```python
from build123d import *

# Parameters (mm, degrees)
SKETCH1_W           = 23
SKETCH1_H           = 104.5
SKETCH1_R           = 2
SKETCH1_R_2         = 5.2
BOSS_EXTRUDE1_DEPTH = 5
SKETCH2_W           = 23
SKETCH2_H           = 20
BOSS_EXTRUDE2_DEPTH = 20
SKETCH3_W           = 23
SKETCH3_H           = 20
BOSS_EXTRUDE3_DEPTH = 5
SKETCH3_3_W         = 100
SKETCH3_3_H         = 20
BOSS_EXTRUDE4_DEPTH = 10
BOSS_EXTRUDE5_DEPTH = 30
BOSS_EXTRUDE6_DEPTH = 30
FILLET1_R           = 10
CUT_EXTRUDE1_DEPTH  = 300
SKETCH6_R           = 13.5
CUT_EXTRUDE2_DEPTH  = 162.5
FILLET5_R           = 3


with BuildPart() as part:
    # Sketch1 → Boss-Extrude1 (new body)
    with BuildSketch(Plane.XY):
        with Locations((0, 30.75)):
            Rectangle(SKETCH1_W, SKETCH1_H)
        with Locations((6.5, 16.5)):
            Circle(SKETCH1_R, mode=Mode.SUBTRACT)
        with Locations((6.5, -16.5)):
            Circle(SKETCH1_R, mode=Mode.SUBTRACT)
        with Locations((0, -12)):
            Circle(SKETCH1_R_2, mode=Mode.SUBTRACT)
        with Locations((-6.5, -16.5)):
            Circle(SKETCH1_R, mode=Mode.SUBTRACT)
        with Locations((-6.5, 16.5)):
            Circle(SKETCH1_R, mode=Mode.SUBTRACT)
    extrude(amount=BOSS_EXTRUDE1_DEPTH)

    # Sketch2 → Boss-Extrude2 (add)
    with BuildSketch(Plane(origin=(0, 0, 0), x_dir=(-1, 0, 0), z_dir=(0, 0, -1))):
        with Locations((0, 73)):
            Rectangle(SKETCH2_W, SKETCH2_H)
    extrude(amount=BOSS_EXTRUDE2_DEPTH)

    # Sketch3 → Boss-Extrude3 (add)
    with BuildSketch(Plane(origin=(0, 0, -20), x_dir=(-1, 0, 0), z_dir=(0, 0, -1))):
        with Locations((0, 73)):
            Rectangle(SKETCH3_W, SKETCH3_H)
    extrude(amount=BOSS_EXTRUDE3_DEPTH)

    # Sketch3<3> → Boss-Extrude4 (add)
    with BuildSketch(Plane(origin=(0, 0, -20), x_dir=(-1, 0, 0), z_dir=(0, 0, -1))):
        with Locations((-61.5, 73)):
            Rectangle(SKETCH3_3_W, SKETCH3_3_H)
        with Locations((61.5, 73)):
            Rectangle(SKETCH3_3_W, SKETCH3_3_H)
    extrude(amount=BOSS_EXTRUDE4_DEPTH)

    # Sketch4 → Boss-Extrude5 (add)
    with BuildSketch(Plane(origin=(111.5, 0, 0), x_dir=(0, 0, -1), z_dir=(1, 0, 0))):
        with BuildLine():
            Line((30, 83), (30, 79.422616289))
            ThreePointArc((30, 79.422616289), (37.803170415, 82.465987391), (44.982034231, 78.151420148))
            Line((44.982034231, 78.151420148), (47.256120501, 79.619062793))
            ThreePointArc((47.256120501, 79.619062793), (39.346969169, 84.978803601), (30, 83))
        make_face()
        with BuildLine():
            ThreePointArc((44.982034231, 67.848579852), (37.803170415, 63.534012609), (30, 66.577383711))
            Line((30, 66.577383711), (30, 63))
            ThreePointArc((30, 63), (39.346969169, 61.021196399), (47.256120501, 66.380937207))
            Line((47.256120501, 66.380937207), (44.982034231, 67.848579852))
        make_face()
    extrude(amount=-BOSS_EXTRUDE5_DEPTH)

    # Sketch5 → Boss-Extrude6 (add)
    with BuildSketch(Plane.ZY.offset(111.5)):
        with BuildLine():
            ThreePointArc((-44.99074033, 78.15631214), (-37.806835348, 82.471571982), (-30, 79.42472441))
            Line((-30, 79.42472441), (-30, 82.742901835))
            ThreePointArc((-30, 82.742901835), (-39.236660525, 84.790740062), (-47.086393259, 79.50952476))
            Line((-47.086393259, 79.50952476), (-44.99074033, 78.15631214))
        make_face()
        with BuildLine():
            Line((-30, 63.257098165), (-30, 66.57527559))
            ThreePointArc((-30, 66.57527559), (-37.806835348, 63.528428018), (-44.99074033, 67.84368786))
            Line((-44.99074033, 67.84368786), (-47.086393259, 66.49047524))
            ThreePointArc((-47.086393259, 66.49047524), (-39.236660525, 61.209259938), (-30, 63.257098165))
        make_face()
    extrude(amount=-BOSS_EXTRUDE6_DEPTH)

    # Fillet1
    fillet1_edges = [part.edges().sort_by_distance(p)[0] for p in [
        (11.5, 73, -20),
        (-11.5, 73, -20),
    ]]
    fillet(fillet1_edges, radius=FILLET1_R)

    # Sketch4<3> → Cut-Extrude1 (cut)
    with BuildSketch(Plane(origin=(111.5, 0, 0), x_dir=(0, 0, -1), z_dir=(1, 0, 0))):
        with BuildLine():
            Line((30, 66.577383711), (30, 73))
            Line((30, 73), (27.5, 73))
            ThreePointArc((27.5, 73), (28.147034395, 69.553987812), (30, 66.577383711))
        make_face()
        with BuildLine():
            Line((27.5, 73), (30, 73))
            Line((30, 73), (30, 79.422616289))
            ThreePointArc((30, 79.422616289), (28.147034395, 76.446012188), (27.5, 73))
        make_face()
    extrude(amount=-CUT_EXTRUDE1_DEPTH, mode=Mode.SUBTRACT)

    # Sketch6 → Cut-Extrude2 (cut)
    with BuildSketch(Plane(origin=(-81.5, 0, 0), x_dir=(0, 0, -1), z_dir=(1, 0, 0))):
        with Locations((37.005416749, 73)):
            Circle(SKETCH6_R)
    extrude(amount=CUT_EXTRUDE2_DEPTH, mode=Mode.SUBTRACT)

    # Fillet5
    # the kernel refuses this fillet: 3 mm, written as the material it takes off along each edge
    with BuildSketch(Plane(origin=(118.086652749, 67.848579852, -44.982034231), x_dir=(0, -0.768500975054365, 0.6398486159557513), z_dir=(-1, 0, 0))) as fillet5_piece_1:
        with BuildLine():
            CenterArc((2.659503922, -2.977998992), FILLET5_R, 96.943270181, 76.113459637)
            Line((-0.318495069, -2.615339366), (-0.378055049, -2.608086174))
            Line((-0.378055049, -2.608086174), (-0.05955998, 0.007253193))
            Line((-0.05955998, 0.007253193), (0.007253193, 0.05955998))
            ThreePointArc((0.007253193, 0.05955998), (1.148422148, -0.009669859), (2.289591104, 0.05955998))
            Line((2.289591104, 0.05955998), (2.296844297, 0))
        make_face()
    extrude(amount=43.173305498, mode=Mode.SUBTRACT)
    with BuildSketch(Plane(origin=(-117.736458127, 67.84368786, -44.99074033), x_dir=(0, -0.5424603966463132, -0.8400813758620795), z_dir=(1, 0, 0))) as fillet5_piece_2:
        with BuildLine():
            CenterArc((2.635643587, -2.996681829), FILLET5_R, 92.695047673, 73.440207037)
            Line((-0.276948751, -2.277789714), (-0.335200598, -2.263411872))
            ThreePointArc((-0.335200598, -2.263411872), (-0.129052561, -1.140040424), (-0.06, 0))
            Line((-0.06, 0), (0, 0.06))
            ThreePointArc((0, 0.06), (1.247291625, 0.06), (2.491762044, 0.059933637))
            Line((2.491762044, 0.059933637), (2.494583251, 0))
        make_face()
    extrude(amount=42.472916254, mode=Mode.SUBTRACT)
    with BuildSketch(Plane(origin=(-117.736458127, 78.15631214, -44.99074033), x_dir=(0, 0.7684660550632233, 0.6398905548729151), z_dir=(1, 0, 0))) as fillet5_piece_3:
        with BuildLine():
            CenterArc((2.656657786, -2.978067915), FILLET5_R, 96.932372645, 73.440207037)
            Line((-0.301090552, -2.476346114), (-0.360245519, -2.466311678))
            ThreePointArc((-0.360245519, -2.466311678), (-0.210106634, -1.230931193), (-0.059561358, 0.007241864))
            Line((-0.059561358, 0.007241864), (0.007241864, 0.059561358))
            ThreePointArc((0.007241864, 0.059561358), (1.147282288, -0.009491202), (2.287322712, 0.059561358))
            Line((2.287322712, 0.059561358), (2.294564576, 0))
        make_face()
    extrude(amount=42.472916254, mode=Mode.SUBTRACT)
    with BuildSketch(Plane(origin=(118.086652749, 78.151420148, -44.982034231), x_dir=(0, 0.5422547524206679, -0.8402141295391314), z_dir=(-1, 0, 0))) as fillet5_piece_4:
        with BuildLine():
            CenterArc((2.6346611, -3), FILLET5_R, 90, 76.113459637)
            Line((-0.277657564, -2.28), (-0.335903938, -2.2656))
            ThreePointArc((-0.335903938, -2.2656), (-0.129229839, -1.141168956), (-0.06, 0))
            Line((-0.06, 0), (0, 0.06))
            Line((0, 0.06), (2.6346611, 0.06))
            Line((2.6346611, 0.06), (2.6346611, 0))
        make_face()
    extrude(amount=43.173305498, mode=Mode.SUBTRACT)


solid = part.part
```
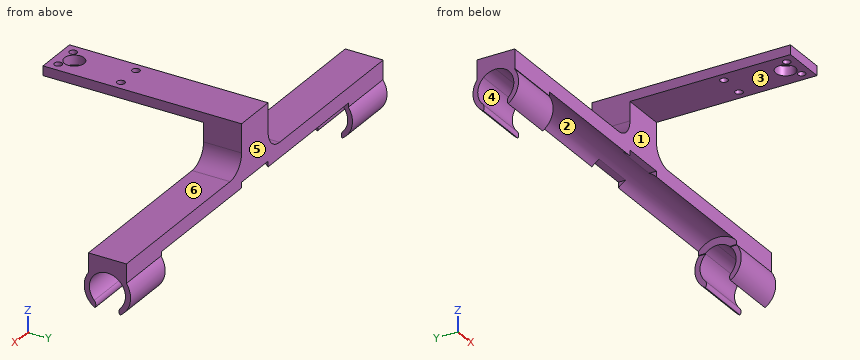
Here's how the part is built. I have some questions about the finished solid (model axes, mm). Face numbers are marked on the shaded views. A direction names the side the tool comes from. Round coordinates to 2 decimals unless told otherwise and drop trailing zeros. Write each loop counter-clockwise with the first axis right and the second up, starting at its lowest first coordinate (ties: lowest second). Pieces come first, ordered by that corner, then holes. Notation, with made-up numbers: M 26.5,81 L 76.5,81 A30 ccw 76.5,112 Z; hole C -20,21.5 d8. An arc over 180 degrees is marked long. Answer as CSV lines item,"result". Start each with the question number.
1. Thinking about a two-plate mould opening in Z: for the marked faces 4, 5 and 6, which applies, released by +Z, released by -Z, zero draft, split by the parting line, or undercut?
2. Suppose I cut it at D-D on y = 36. Write out the boundary of the cut face in (x, z).
3. Suppose I cut it at C-C on x = 86. Write out the boundary of the cut face in (y, z).
4. Suppose I cut it at A-A on y = -12. Write out the boundary of the cut face in (x, z), then the cut area to 3 significant figures.
5. Suppose I cut it at B-B on x = 0. Write out the boundary of the cut face in (y, z), then the cut area to 3 significant figures.
6. I'm going to push flat-ended pins straight in: pin 1 Ø1.9 at (x, y) = (1, 82) entering from -Z; pin 2 Ø7.5 at (y, z) = (32, -1.5) entering from +X; pin 3 Ø5 at (x, y) = (-6.5, 16.5) entering from -Z. Where does each tip first touch, or does it pass through?
7. I need wall thicknesses on probe 1 along Y at (x, z) = (6.5, 2.6); probe 2 along Y at (x, z) = (6, 2); probe 3 along X at (y, z) = (-16, 3). Which ranges of each line are inside material? Lowest first, please.
8. On a 3-axis mill with a long thin cutter (end or side, diameter ignored), from which of +Z, -Z, +X, -X, +Y, -Y can I reach the whole of each face in a straight line? I mean the marked faces 1, 2 and 3. Say none if no direction works.
Check result:
1,face 4,"undercut"
1,face 5,"zero draft"
1,face 6,"released by +Z"
2,outline,"M -11.5,0 L 11.5,0 L 11.5,5 L -11.5,5 Z"
3,outline,"M 63,-30 A12.21 ccw 66.38,-47.26 L 66.42,-47.2 A3 ccw 66.08,-43.51 A9.5 cw long 79.92,-43.51 A3 ccw 79.58,-47.2 L 79.62,-47.26 A12.21 ccw 83,-30 L 83,-20 L 63,-20 Z"
4,outline,"M -11.5,0 L -5.2,0 L -5.2,5 L -11.5,5 Z; M 5.2,0 L 11.5,0 L 11.5,5 L 5.2,5 Z"
4,area,"63.0 mm2"
5,outline,"M -21.5,0 L -17.2,0 L -17.2,5 L -21.5,5 Z; M -6.8,0 L 63,0 L 63,-25 L 66.83,-25 A13.5 cw 79.17,-25 L 83,-25 L 83,5 L -6.8,5 Z"
5,area,"958 mm2"
6,pin 1,"stops at z = -25"
6,pin 2,"stops at x = 11.5"
6,pin 3,"stops at z = 0"
7,probe 1,"y = -21.5 to -18.5, -14.5 to 14.5, 18.5 to 83"
7,probe 2,"y = -21.5 to -18.44, -14.56 to 14.56, 18.44 to 83"
7,probe 3,"x = -11.5 to -8.44, -4.56 to -3.32, 3.32 to 4.56, 8.44 to 11.5"
8,face 1,"+X, -X, -Y"
8,face 2,"-Z"
8,face 3,"-Z, +X, -X, -Y"
